Source: three-view drawing plus pictorial views. Frame: mm from the lowest corner of the part. A direction names the side the tool comes from. Coordinates: 2 decimals unless noted, no trailing zeros. Loops run counter-clockwise (first coordinate to the right, second up) from the corner with the lowest first, then second, coordinate; pieces in that order, holes last. Notation, with made-up numbers: (6, 2) - (28, 2) arc R22 ccw to (28, 30) - close; hole circle Ø3 at (21, -39.5). An arc over 180 degrees is marked (long way). Answer as CSV lines item,"result". Start each with the question number.
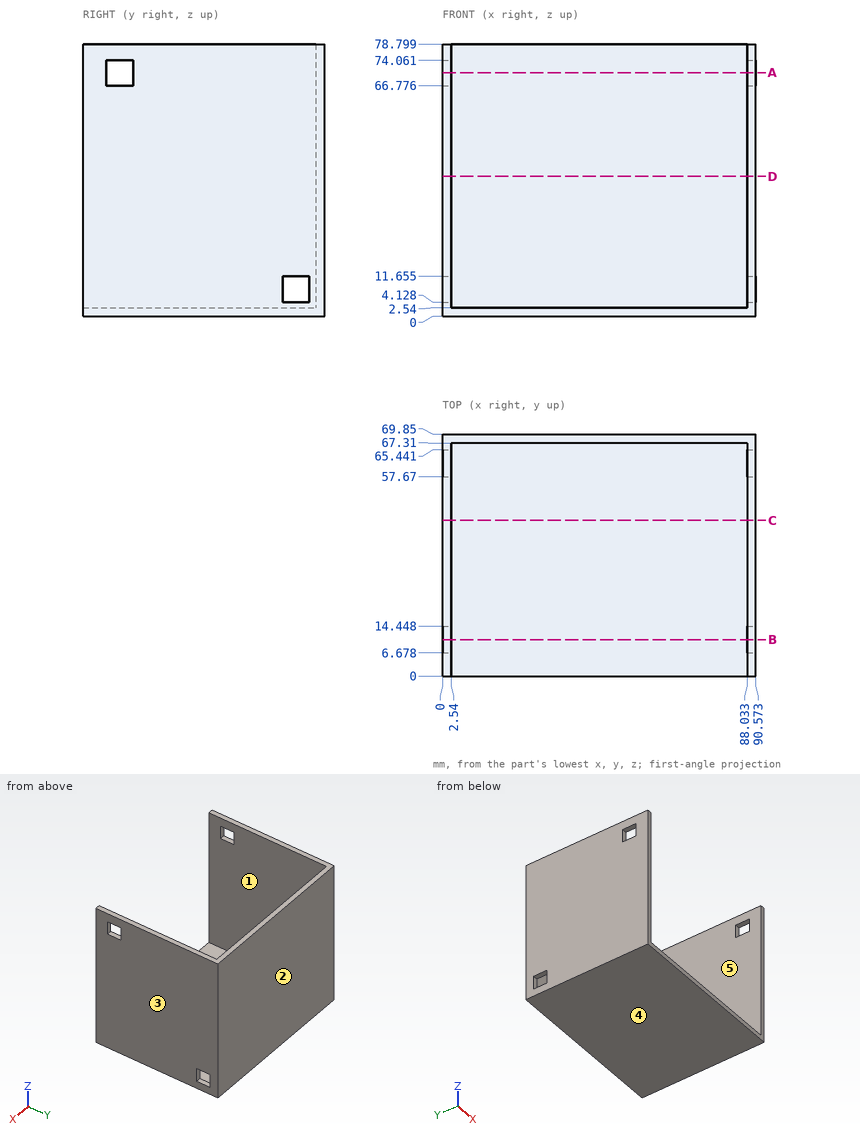
Item 1: Section query B-B, the plane y = 10.5. Output: boundary loops of the cut face in (x, z).
Item 2: Material intervals for probe 1 along X at (y, z) = (29.5, 58); probe 2 along Y at (x, z) = (44, 56); probe 3 along Z at (x, y) = (53, 62), sorted ascending.
Item 3: Draft query along X for the marked faces 1, 2 and 3. Return one class per face: pulls with the +X half, pulls with the -X half, needs draft (parallel to the pull), parting line crosses it, or undercut.
Item 4: Set-up query: the marked faces 4 and 5. Return all of +Z, -Z, +X, -X, +Y, -Y with unobstructed straight access to the full face (end or side cutting, diameter ignored); none if empty.
Item 5: Section query D-D, the plane z = 40.5. Output: boundary loops of the cut face in (x, y).
Item 6: Section query C-C, the plane y = 45. Output: boundary loops of the cut face in (x, z).
Item 7: Contact query for flat-ended pins moving along their axis: P1, Ø23, axis at x = 64.5, z = 47.5, coming from the -Y side; P2, Ø1.3, axis at x = 1, z = 7.5, coming from the -Y side. Output: stop coordinate, or through.
Item 8: Section query A-A, the plane z = 70.5. Output: boundary loops of the cut face in (x, y).
Response values:
1,outline,"(0, 0) - (90.57, 0) - (90.57, 66.78) - (88.03, 66.78) - (88.03, 2.54) - (2.54, 2.54) - (2.54, 66.78) - (0, 66.78) - close; (0, 74.06) - (2.54, 74.06) - (2.54, 78.8) - (0, 78.8) - close; (88.03, 74.06) - (90.57, 74.06) - (90.57, 78.8) - (88.03, 78.8) - close"
2,probe 1,"x = 0 to 2.54, 88.03 to 90.57"
2,probe 2,"y = 67.31 to 69.85"
2,probe 3,"z = 0 to 2.54"
3,face 1,"undercut"
3,face 2,"needs draft"
3,face 3,"pulls with the +X half"
4,face 4,"-Z, +X, -X, +Y, -Y"
4,face 5,"+Z, -Y"
5,outline,"(0, 0) - (2.54, 0) - (2.54, 67.31) - (88.03, 67.31) - (88.03, 0) - (90.57, 0) - (90.57, 69.85) - (0, 69.85) - close"
6,outline,"(0, 0) - (90.57, 0) - (90.57, 78.8) - (88.03, 78.8) - (88.03, 2.54) - (2.54, 2.54) - (2.54, 78.8) - (0, 78.8) - close"
7,P1,"stops at y = 67.31"
7,P2,"stops at y = 0"
8,outline,"(0, 0) - (2.54, 0) - (2.54, 6.68) - (0, 6.68) - close; (0, 14.45) - (2.54, 14.45) - (2.54, 67.31) - (88.03, 67.31) - (88.03, 14.45) - (90.57, 14.45) - (90.57, 69.85) - (0, 69.85) - close; (88.03, 0) - (90.57, 0) - (90.57, 6.68) - (88.03, 6.68) - close"
